The drawing under review shows one solid part. Ordinate dimensions are in mm from its lowest x, y, z. A direction names the side the tool comes from. Give positions to 0.01 mm unless a question says otherwise; leave off trailing zeros. Loops run counter-clockwise (first coordinate to the right, second up) from the corner with the lowest first, then second, coordinate; pieces in that order, holes last. Notation, with made-up numbers: M 45.25,-28 L 64.25,-28 A31 ccw 64.25,2 Z; hole C 0,59.25 d8. An arc over 180 degrees is marked long. Put each result on its own line as item: value. Start each with the question number.
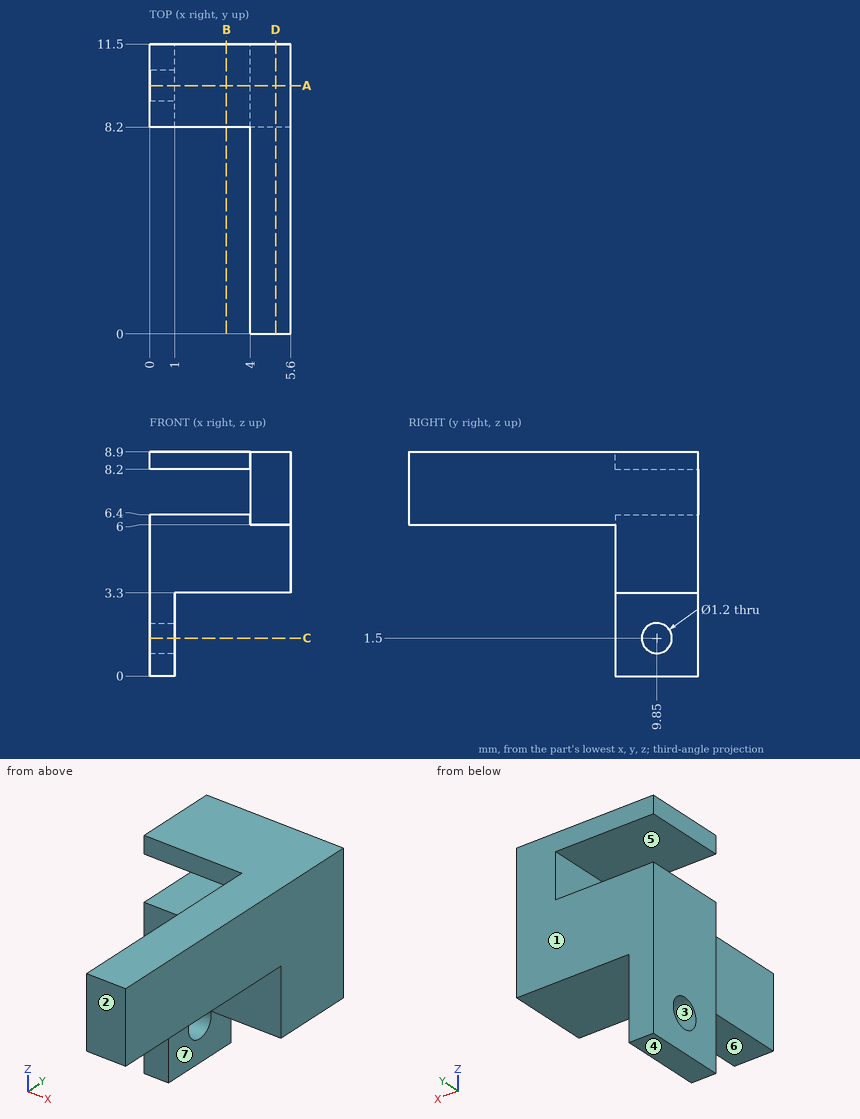
(1) We need section D-D, the plane x = 5. Write out the cut boundary in (y, z).
(2) We need section A-A, the plane y = 9.85. Write out the cut boundary in (x, z), plus the area to 3 significant figures.
(3) Draft analysis for pull direction Y (two halves, no side actions). For the marked faces 1, 2 and 3, state which applies: +Y half, -Y half, draft (parallel to the pull), parting line (faces both ways), or undercut.
(4) Insertion check: pin 1 (1 mm diameter, centred on y = 9.5, z = 1.5, fed in from +X); pin 2 (1.7 mm diameter, centred on x = 2, y = 10, fed in from -Z); pin 3 (1.7 mm diameter, centred on x = 3, z = 3.5, fed in from -Y). Each pin has a flat end and moves straight along its axis. Give the tip position at first contact, or say it passes through.
(5) We need section B-B, the plane x = 3.05. Write out the cut boundary in (y, z).
(6) We need section C-C, the plane z = 1.5. Write out the cut boundary in (x, y).
(7) To check wall thickness, follow L1, parallel to Z at x = 0.3, y = 9.85; L2, parallel to Z at x = 1.9, y = 9.5; L3, parallel to Z at x = 4.6, y = 7.75. State the ranges of each line that lie inside material, in increasing order. Write a range as [from, to].
(8) For the marked faces 4, 5, 6 and 7, list the 3-axis set-ups (+Z, -Z, +X, -X, +Y, -Y) from which the entire face can be reached by the end or side of a thin tool; tool diameter is ignored.
Check sheet entries:
1. outline: M 0,6 L 8.2,6 L 8.2,3.3 L 11.5,3.3 L 11.5,8.9 L 0,8.9 Z
2. outline: M 0,0 L 1,0 L 1,0.9 L 0,0.9 Z; M 0,2.1 L 1,2.1 L 1,3.3 L 5.6,3.3 L 5.6,8.9 L 0,8.9 L 0,8.2 L 4,8.2 L 4,6.4 L 0,6.4 Z
2. area: 26.3 mm²
3. face 1: +Y half
3. face 2: -Y half
3. face 3: undercut
4. pin 1: stops at x = 1
4. pin 2: stops at z = 3.3
4. pin 3: stops at y = 8.2
5. outline: M 8.2,3.3 L 11.5,3.3 L 11.5,6.4 L 8.2,6.4 Z; M 8.2,8.2 L 11.5,8.2 L 11.5,8.9 L 8.2,8.9 Z
6. outline: M 0,8.2 L 1,8.2 L 1,9.25 L 0,9.25 Z; M 0,10.45 L 1,10.45 L 1,11.5 L 0,11.5 Z
7. L1: z = [0, 0.9], [2.1, 6.4], [8.2, 8.9]
7. L2: z = [3.3, 6.4], [8.2, 8.9]
7. L3: z = [6, 8.9]
8. face 4: -Z, +X, -X, +Y, -Y
8. face 5: -X, +Y, -Y
8. face 6: -Z, +X, -X, -Y
8. face 7: -Z, +X, +Y, -Y
